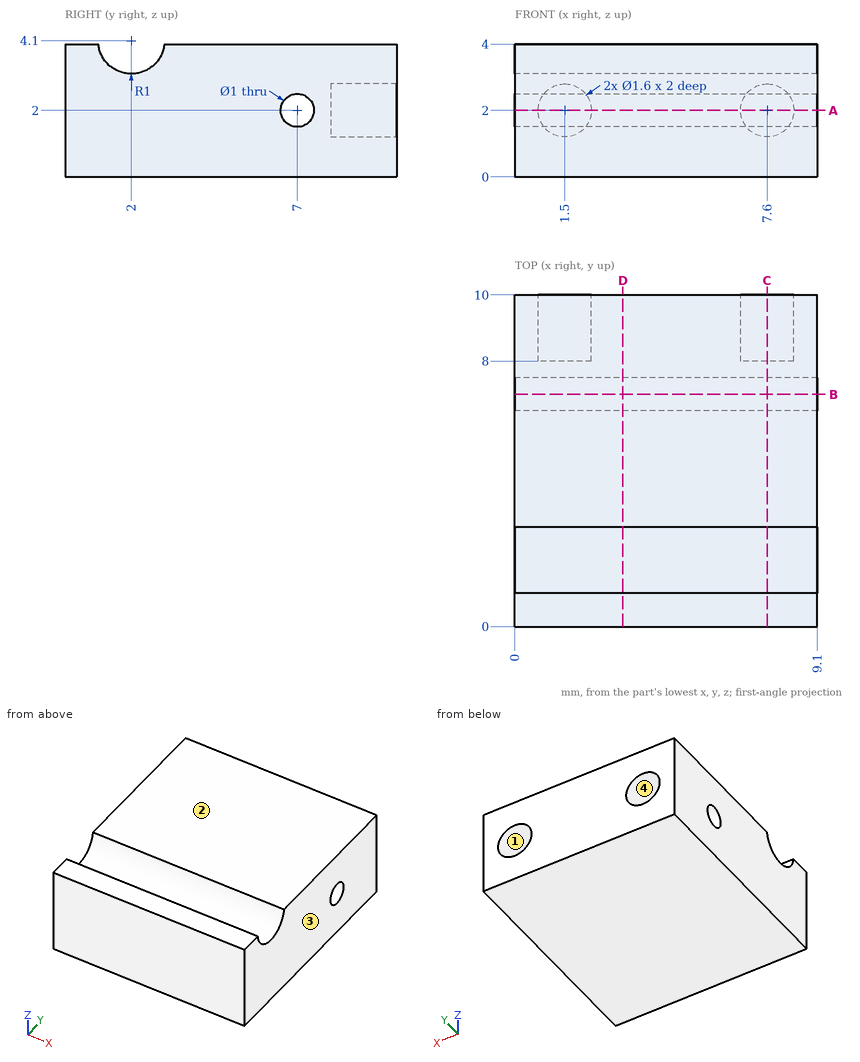
Design review of the part shown in the three views and the two pictorial views. Dimensions are in mm from the part's minimum x, y and z. Coordinates: 2 decimals unless noted, no trailing zeros. Loops run counter-clockwise (first coordinate to the right, second up) from the corner with the lowest first, then second, coordinate; pieces in that order, holes last. Notation, with made-up numbers: M 31,74 L 74,74 A7 cw 74,79 Z; hole C -34,39.5 d2. An arc over 180 degrees is marked long. One line per question, with ' | ' between items.
(1) Draft analysis for pull direction X (two halves, no side actions). For the marked faces 1, 2, 3 and 4, state which applies: released by +X, released by -X, zero draft, split by the parting line, or undercut.
Filled in:
face 1: undercut | face 2: zero draft | face 3: released by +X | face 4: undercut
(2) We need section D-D (x = 3.25). Give the boundary of the cut face in (y, z).
Filled in:
outline: M 0,0 L 10,0 L 10,4 L 2.99,4 A1 cw 1.01,4 L 0,4 Z; hole C 7,2 d1
(3) We need section B-B (y = 7). Give the boundary of the cut face in (x, z), and give its area (3 significant figures).
Filled in:
outline: M 0,0 L 9.1,0 L 9.1,1.5 L 0,1.5 Z; M 0,2.5 L 9.1,2.5 L 9.1,4 L 0,4 Z | area: 27.3 mm^2
(4) We need section A-A (z = 2). Give the boundary of the cut face in (x, y), and give its area (3 significant figures).
Filled in:
outline: M 0,0 L 9.1,0 L 9.1,6.5 L 0,6.5 Z; M 0,7.5 L 9.1,7.5 L 9.1,10 L 8.4,10 L 8.4,8 L 6.8,8 L 6.8,10 L 2.3,10 L 2.3,8 L 0.7,8 L 0.7,10 L 0,10 Z | area: 75.5 mm^2
(5) For pin 1 Ø1 at (y, z) = (6, 2) entering from -X; pin 2 Ø0.5 at (x, z) = (7.5, 2.5) entering from +Y, all flat-tipped, find the tip position at first contact; note any pin that passes through.
Filled in:
pin 1: stops at x = 0 | pin 2: stops at y = 8
(6) Wall thickness on probe 1 along X at (y, z) = (9.3, 2); probe 2 along X at (y, z) = (8.5, 2.7); probe 3 along Y at (x, z) = (5, 2.05): over which ranges is each line inside the solid? List them lowest first.
Filled in:
probe 1: x = 0 to 0.7, 2.3 to 6.8, 8.4 to 9.1 | probe 2: x = 0 to 1.11, 1.89 to 7.21, 7.99 to 9.1 | probe 3: y = 0 to 6.5, 7.5 to 10
(7) We need section C-C (x = 7.6). Give the boundary of the cut face in (y, z), and give its area (3 significant figures).
Filled in:
outline: M 0,0 L 10,0 L 10,1.2 L 8,1.2 L 8,2.8 L 10,2.8 L 10,4 L 2.99,4 A1 cw 1.01,4 L 0,4 Z; hole C 7,2 d1 | area: 34.6 mm^2
